Design review of the part built by this model. Coordinates are the model's own, in mm. A direction names the side the tool comes from. Coordinates: 2 decimals unless noted, no trailing zeros. Order: outer loops, then holes, each group sorted by start corner. A loop starts at its lowest first (then second) coordinate and runs counter-clockwise, first axis right, second up. Notation, with made-up numbers: (29.5, 51.25) -> (75.5, 51.25) arc R19 ccw to (75.5, 80.25) -> close; hole circle Ø3 at (69, 32). An arc over 180 degrees is marked (long way). Use a Markdown table: item, result. Add a question column.
Q1. The part is to be moulded in two halves that separate along X. For faces 3 (the face through (0, -6, -9.525)), 4 (the face through (-0.86, -6.261, -3.874)), 5 (the face through (-9.525, -6, 0)), say which applies: pulls with the +X half, pulls with the -X half, needs draft (parallel to the pull), parting line crosses it, or undercut.
Q2. Machinability: for faces 1 (the face through (4, -12.7, -2)), 2 (the face through (-0.133, -6.844, 9.017)), which of the approach directions +Z, -Z, +X, -X, +Y, -Y give a long, thin tool a straight path to every point of the face, cutting with its end or side? Answer none if there is none.
Q3. Wall thickness on probe 1 along Z at (x, y) = (0, -3.5) (3 decimals); probe 2 along X at (y, z) = (-10.5, 1.5) (3 decimals): over which ranges is each line inside the solid? List them lowest first.
Q4. Add section B-B (y = -7). State the section outline as (x, z) points (1 decimal), then the cut area to 3 significant figures.
Q5. Add section A-A (y = -11). State the section outline as (x, z) points (1 decimal).
from build123d import *

# Parameters (mm, degrees)
F0_R     = 3.96875
F1_DEPTH = 12.7
F5_DEPTH = 127


with BuildPart() as f1:
    # F0 (on Front) → F1 (new body)
    with BuildSketch(Plane.XZ):
        with BuildLine():
            ThreePointArc((0, -9.525), (6.7351920908, -6.7351920908), (9.525, 0))
            ThreePointArc((9.525, 0), (6.7351920908, 6.7351920908), (0, 9.525))
            ThreePointArc((0, 9.525), (-6.7351920908, 6.7351920908), (-9.525, 0))
            ThreePointArc((-9.525, 0), (-6.7351920908, -6.7351920908), (0, -9.525))
        make_face()
        Circle(F0_R, mode=Mode.SUBTRACT)
        with BuildLine():
            Line((9.525, -9.525), (9.525, 0))
            ThreePointArc((9.525, 0), (6.7351920908, -6.7351920908), (0, -9.525))
            Line((0, -9.525), (9.525, -9.525))
        make_face()
        with BuildLine():
            ThreePointArc((0, 9.525), (6.7351920908, 6.7351920908), (9.525, 0))
            Line((9.525, 0), (9.525, 9.525))
            Line((9.525, 9.525), (0, 9.525))
        make_face()
        with BuildLine():
            ThreePointArc((-9.525, 0), (-6.7351920908, 6.7351920908), (0, 9.525))
            Line((0, 9.525), (-9.525, 9.525))
            Line((-9.525, 9.525), (-9.525, 0))
        make_face()
        with BuildLine():
            Line((-9.525, -9.525), (0, -9.525))
            ThreePointArc((0, -9.525), (-6.7351920908, -6.7351920908), (-9.525, 0))
            Line((-9.525, 0), (-9.525, -9.525))
        make_face()
    extrude(amount=F1_DEPTH)

    # F4 (on face) → F5 (cut)
    with BuildSketch(Plane(origin=(-9.525, 0, 0), x_dir=(0, -1, 0), z_dir=(-1, 0, 0))):
        Polygon((3.6136890898, 11.2591073548), (6.35, 8.5227964446), (9.0863109102, 11.2591073548), align=None)
    extrude(amount=-F5_DEPTH, mode=Mode.SUBTRACT)

    # F6 (on face) → F7 (revolve, cut)
    with BuildSketch(Plane.YZ):
        Polygon((-12.7, 15.6255830079), (-12.7, 9.525), (-11.0653537097, 15.6255830079), align=None)
    revolve(axis=Axis((0, 0, 0), (0, 1, 0)), mode=Mode.SUBTRACT)

    # F8 (on face) → F9 (revolve, cut)
    with BuildSketch(Plane.YZ):
        Polygon((-1.1722899654, 13.910143229), (0, 9.5350975171), (0, 13.910143229), align=None)
    revolve(axis=Axis((0, 0, 0), (0, -1, 0)), mode=Mode.SUBTRACT)


solid = f1.part
Established:
| question | item | result |
|---|---|---|
| 1 | face 3 | needs draft |
| 1 | face 4 | undercut |
| 1 | face 5 | pulls with the -X half |
| 2 | face 1 | +Z, -Z, +X, -X, -Y |
| 2 | face 2 | +Z, +X, -X |
| 3 | probe 1 | -9.525 to -3.969, 3.969 to 9.525 |
| 3 | probe 2 | -9.525 to -3.674, 3.674 to 9.525 |
| 4 | outline | (-9.5, -9.5) -> (9.5, -9.5) -> (9.5, 9.2) -> (-9.5, 9.2) -> close; hole circle Ø7.9 at (0, 0) |
| 4 | area | 307 mm^2 |
| 5 | outline | (-9.5, -9.5) -> (9.5, -9.5) -> (9.5, 9.5) -> (-9.5, 9.5) -> close; hole circle Ø7.9 at (0, 0) |
